Geometry: see drawing. Coordinates: mm, zero at the bounding-box minimum. Coordinates: 2 decimals unless noted, no trailing zeros. Write each loop counter-clockwise with the first axis right and the second up, starting at its lowest first coordinate (ties: lowest second). Pieces come first, ordered by that corner, then holes. Notation, with made-up numbers: (49.25, -2.5) -> (85.25, -2.5) arc R32 cw to (85.25, 24.5) -> close; hole circle Ø2 at (-30.5, 52). An arc over 180 degrees is marked (long way). Answer as a JSON object with one key per item and string values. Group by question number.
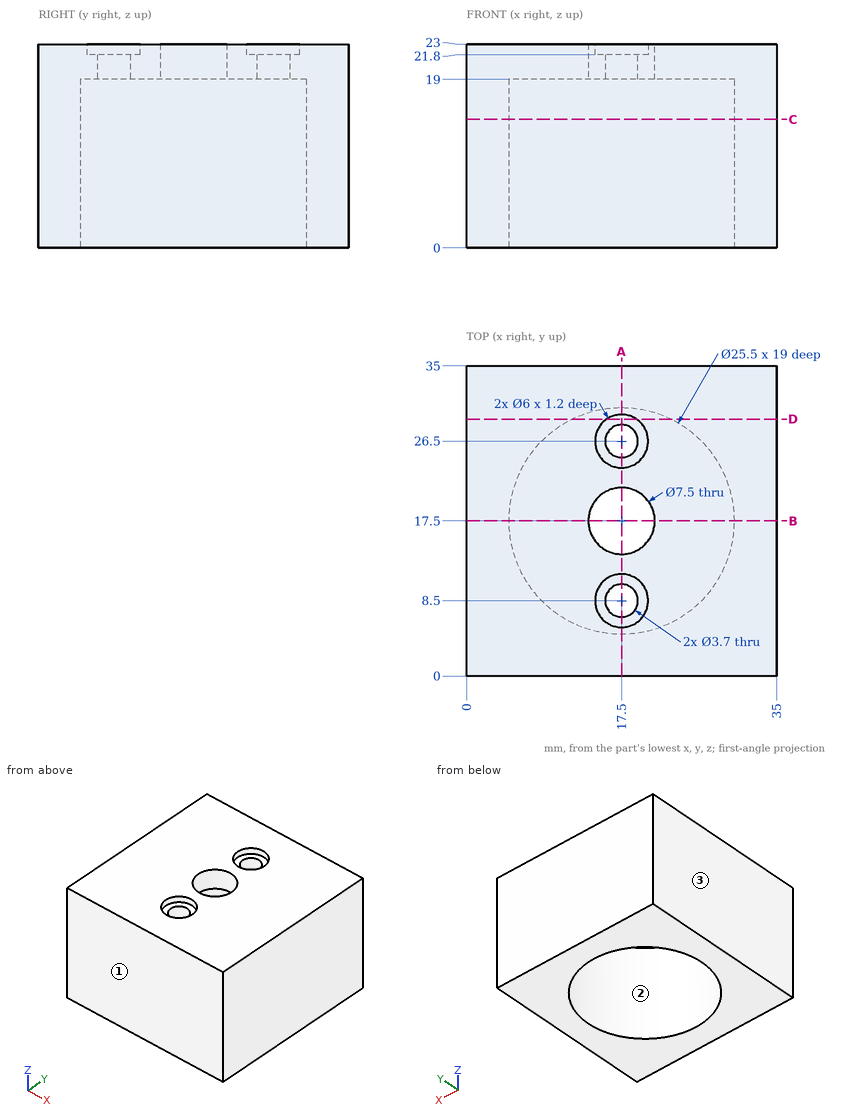
Item 1: Section D-D on y = 29. Output: boundary loops of the cut face in (x, z), then the cut area to 3 significant figures.
Item 2: Section A-A on x = 17.5. Output: boundary loops of the cut face in (y, z).
Item 3: Ray query, L1, parallel to Y at x = 17.5, z = 19.8; L2, parallel to Y at x = 17.5, z = 21.85; L3, parallel to Z at x = 21, y = 29.5. Return the intervals inside material, ascending. Write a range as [from, to].
Item 4: Section C-C on z = 14.5. Output: boundary loops of the cut face in (x, y).
Item 5: Section B-B on y = 17.5. Output: boundary loops of the cut face in (x, z), then the cut area to 4 significant figures.
Item 6: Mould query, pull axis Y, two halves, no side actions, for the marked faces 1, 2 and 3. Classes: +Y half, -Y half, draft (parallel to the pull), parting line (faces both ways), or undercut.
Item 7: Contact query for flat-ended pins moving along their axis: pin 1 (5 mm diameter, centred on x = 17.5, y = 26.5, fed in from +Z); pin 2 (4.5 mm diameter, centred on x = 17.5, y = 17.5, fed in from -Z); pin 3 (5 mm diameter, centred on x = 17, y = 14.5, fed in from -Z). Output: stop coordinate, or through.
Answer sheet:
{
 "1": {"outline": "(0, 0) -> (11.99, 0) -> (11.99, 19) -> (23.01, 19) -> (23.01, 0) -> (35, 0) -> (35, 23) -> (19.16, 23) -> (19.16, 21.8) -> (15.84, 21.8) -> (15.84, 23) -> (0, 23) -> close", "area": "592 mm^2"},
 "2": {"outline": "(0, 0) -> (4.75, 0) -> (4.75, 19) -> (6.65, 19) -> (6.65, 21.8) -> (5.5, 21.8) -> (5.5, 23) -> (0, 23) -> close; (10.35, 19) -> (13.75, 19) -> (13.75, 23) -> (11.5, 23) -> (11.5, 21.8) -> (10.35, 21.8) -> close; (21.25, 19) -> (24.65, 19) -> (24.65, 21.8) -> (23.5, 21.8) -> (23.5, 23) -> (21.25, 23) -> close; (28.35, 19) -> (30.25, 19) -> (30.25, 0) -> (35, 0) -> (35, 23) -> (29.5, 23) -> (29.5, 21.8) -> (28.35, 21.8) -> close"},
 "3": {"L1": "y = [0, 6.65], [10.35, 13.75], [21.25, 24.65], [28.35, 35]", "L2": "y = [0, 5.5], [11.5, 13.75], [21.25, 23.5], [29.5, 35]", "L3": "z = [19, 23]"},
 "4": {"outline": "(0, 0) -> (35, 0) -> (35, 35) -> (0, 35) -> close; hole circle Ø25.5 at (17.5, 17.5)"},
 "5": {"outline": "(0, 0) -> (4.75, 0) -> (4.75, 19) -> (13.75, 19) -> (13.75, 23) -> (0, 23) -> close; (21.25, 19) -> (30.25, 19) -> (30.25, 0) -> (35, 0) -> (35, 23) -> (21.25, 23) -> close", "area": "290.5 mm^2"},
 "6": {"face 1": "-Y half", "face 2": "undercut", "face 3": "draft"},
 "7": {"pin 1": "stops at z = 21.8", "pin 2": "passes through", "pin 3": "stops at z = 19"}
}
